For this review, take the finished solid that the model builds, in its own axes (mm). Give positions to 0.01 mm unless a question says otherwise; leave off trailing zeros. Loops run counter-clockwise (first coordinate to the right, second up) from the corner with the lowest first, then second, coordinate; pieces in that order, holes last. Notation, with made-up numbers: (14.25, 42) - (39.25, 42) arc R11 ccw to (39.25, 46) - close; hole circle Ø8 at (-2, -10.5). An arc over 180 degrees is marked (long way). Put each result on its own line as item: value.
from build123d import *

# Parameters (mm, degrees)
BOSS_EXTRUDE1_DEPTH = 0.42
SKETCH2_R           = 2.05
CUT_EXTRUDE1_DEPTH  = 76.213334038
FILLET1_R           = 10
FILLET2_R           = 0.5
FILLET3_R           = 2
FILLET4_R           = 2
FILLET5_R           = 0.5
FILLET6_R           = 2


with BuildPart() as part:
    # Sketch1 → Boss-Extrude1 (new, symmetric)
    with BuildSketch(Plane(origin=(0, 0, 0), x_dir=(1, 0, 0), z_dir=(0, 1, 0))):
        with BuildLine():
            Line((2.5, 68), (2.5, 74.5))
            Line((2.5, 74.5), (10.3, 74.5))
            Line((10.3, 74.5), (10.3, 68))
            add(Edge.make_bspline(
                [(10.3, 68), (8.714398617, 49.11082539), (11.816891749, 28.482557039), (8.564530207, 15.25)],
                knots=[0, 0, 0, 0, 1, 1, 1, 1], degree=3))
            Line((8.564530207, 15.25), (0, 0))
            Line((0, 0), (-8, 15.25))
            Line((-8, 15.25), (0.382846681, 27.081224853))
            add(Edge.make_bspline(
                [(7.3, 38), (7.400709228, 32.674514217), (6.147076675, 31.910033807), (0.382846681, 27.081224853)],
                knots=[0, 0, 0, 0, 1, 1, 1, 1], degree=3))
            Line((7.3, 38), (7.3, 59))
            add(Edge.make_bspline(
                [(2.5, 68), (6.364741582, 67.576851124), (7.3, 59)],
                knots=[0, 0, 0, 1, 1, 1], degree=2))
        make_face()
    extrude(amount=BOSS_EXTRUDE1_DEPTH, both=True)

    # Sketch2 → Cut-Extrude1 (cut, through all)
    with BuildSketch(Plane(origin=(0, 0.42, 0), x_dir=(1, 0, 0), z_dir=(0, 1, 0))):
        with Locations(Location((6.75, 70.6, 0), (0, 0, 270))):
            Circle(SKETCH2_R)
    extrude(amount=-CUT_EXTRUDE1_DEPTH, mode=Mode.SUBTRACT)

    # Fillet1
    fillet1_edges = [part.edges().sort_by_distance(p)[0] for p in [
        (8.564530207, -0.21, -15.25),
        (0.382846681, -0.21, -27.081224853),
    ]]
    fillet(fillet1_edges, radius=FILLET1_R)

    # Fillet2
    fillet2_edges = [part.edges().sort_by_distance(p)[0] for p in [
        (2.5, -0.21, -68),
    ]]
    fillet(fillet2_edges, radius=FILLET2_R)

    # Fillet3
    fillet3_edges = [part.edges().sort_by_distance(p)[0] for p in [
        (2.5, 0, -74.5),
        (10.3, 0, -74.5),
    ]]
    fillet(fillet3_edges, radius=FILLET3_R)

    # Fillet4
    fillet4_edges = [part.edges().sort_by_distance(p)[0] for p in [
        (-8, 0, -15.25),
    ]]
    fillet(fillet4_edges, radius=FILLET4_R)

    # Fillet5
    fillet5_edges = [part.edges().sort_by_distance(p)[0] for p in [
        (0, 0, 0),
    ]]
    fillet(fillet5_edges, radius=FILLET5_R)

    # Fillet6
    # the kernel refuses this fillet: 2 mm, written as the material it adds along each edge
    with BuildSketch(Plane(origin=(7.3, 0, -59), x_dir=(0, 0, 1), z_dir=(0, -1, 0))) as fillet6_piece_1:
        with BuildLine():
            CenterArc((0.110157954, 2), FILLET6_R, 263.610060097, 6.389939903)
            ThreePointArc((-0.112430932, 0.012425048), (-0.056219986, 0.006171626), (0, 0))
            Line((0, 0), (0.110157954, 0))
        make_face()
    extrude(amount=0.42)
    with BuildSketch(Plane(origin=(7.3, 0, -59), x_dir=(0, 0, 1), z_dir=(0, 1, 0))) as fillet6_piece_2:
        with BuildLine():
            CenterArc((0.110157954, -2), FILLET6_R, 90, 6.389939903)
            ThreePointArc((-0.112430932, -0.012425048), (-0.056219986, -0.006171626), (0, 0))
            Line((0, 0), (0.110157954, 0))
        make_face()
    extrude(amount=0.42)
    # the kernel refuses this fillet: 2 mm, written as the material it takes off along each edge
    with BuildSketch(Plane(origin=(7.3, 0.046586814, -38), x_dir=(0, 0, -1), z_dir=(0, -1, 0))) as fillet6_2_piece_1:
        with BuildLine():
            CenterArc((0.018634726, 2), FILLET6_R, 268.947653116, 1.052346884)
            ThreePointArc((-0.018097045, 0.000337334), (-0.0090485, 0.000169892), (0, 0))
            Line((0, 0), (0.018634726, 0))
        make_face()
    extrude(amount=0.513173628, mode=Mode.SUBTRACT)
    with BuildSketch(Plane(origin=(10.3, 0, -68), x_dir=(-0.08328041944419425, 0, 0.9965261520588404), z_dir=(0, -1, 0))) as fillet6_2_piece_2:
        with BuildLine():
            CenterArc((0.083426948, 1.999999864), FILLET6_R, 265.222850471, 4.756036045)
            Line((-0.083133891, 0.00694756), (0, 0))
            ThreePointArc((0, 0), (0.041344974, 7.623e-06), (0.082689948, 0))
        make_face()
    extrude(amount=0.628559231, mode=Mode.SUBTRACT)
    with BuildSketch(Plane(origin=(10.3, 0, -68), x_dir=(-0.08328041944419425, 0, 0.9965261520588404), z_dir=(0, 1, 0))) as fillet6_2_piece_3:
        with BuildLine():
            CenterArc((0.083426948, -1.999999864), FILLET6_R, 90.021113485, 4.756036045)
            Line((-0.083133891, -0.00694756), (0, 0))
            ThreePointArc((0, 0), (0.041344974, -7.623e-06), (0.082689948, 0))
        make_face()
    extrude(amount=0.628559231, mode=Mode.SUBTRACT)


solid = part.part
1) Wall thickness on line 1 (X direction, y = 0.2, z = -70.6); line 2 (Z direction, x = 3.5, y = 0.25); line 3 (X direction, y = 0.1, z = -63): over which ranges is each line inside the solid? List them lowest first.
Geometry check:
line 1: x = 2.5 to 4.7, 8.8 to 10.3
line 2: z = -74.23 to -67.73, -29.71 to -6.23
line 3: x = 6.59 to 9.98
2) Take a section at B-B on z = -6. State the section outline as (x, y) points.
Geometry check:
outline: (-3.15, -0.42) - (3.37, -0.42) - (3.37, 0.42) - (-3.15, 0.42) - close
3) Take a section at A-A on z = -70.6. State the section outline as (x, y) points, and give its area (3 significant figures).
Geometry check:
outline: (2.5, -0.42) - (4.7, -0.42) - (4.7, 0.42) - (2.5, 0.42) - close; (8.8, -0.42) - (10.3, -0.42) - (10.3, 0.42) - (8.8, 0.42) - close
area: 3.11 mm²
